```python
from build123d import *

# Parameters (mm, degrees)
SKETCH001_W        = 48
SKETCH001_H        = 51
SKETCH001_R        = 3.5
SKETCH001_R_2      = 2.25
PAD_DEPTH          = 3.41
SKETCH002_W        = 51
SKETCH002_H        = 45
PAD001_DEPTH       = 2.17
PAD002_DEPTH       = 25.56
POLARPATTERN_COUNT = 4
PAD003_DEPTH       = 3
CHAMFER_SIZE       = 2.8
FILLET_R           = 6
FILLET001_R        = 22


with BuildPart() as part:
    # Sketch001 → Pad (new body)
    with BuildSketch(Plane.XY):
        Rectangle(SKETCH001_W, SKETCH001_H)
        with Locations((-18.5, 17)):
            Circle(SKETCH001_R, mode=Mode.SUBTRACT)
        with Locations((15, 17)):
            Circle(SKETCH001_R_2, mode=Mode.SUBTRACT)
        with Locations((-18.5, -17)):
            Circle(SKETCH001_R, mode=Mode.SUBTRACT)
        with Locations((15, -17)):
            Circle(SKETCH001_R_2, mode=Mode.SUBTRACT)
    extrude(amount=PAD_DEPTH)

    # Sketch002 → Pad001 (join)
    with BuildSketch(Plane(origin=(-24, 0, 0), x_dir=(0, -1, 0), z_dir=(-1, 0, 0))):
        with Locations((0, 22.5)):
            Rectangle(SKETCH002_W, SKETCH002_H)
    extrude(amount=PAD001_DEPTH)

    # Sketch → Pad002 (join)
    with BuildSketch(Plane(origin=(-26.17, 0, 26), x_dir=(0, -1, 0), z_dir=(-1, 0, 0))):
        with BuildLine():
            ThreePointArc((16.420739, 4.399924), (12.028925, 12.0127), (4.422085, 16.414785))
            ThreePointArc((3.11174, 17.647793), (3.652144, 16.909322), (4.422085, 16.414785))
            ThreePointArc((3.11174, 17.647793), (2.656255, 18.151957), (2, 18.327959))
            ThreePointArc((2, 18.327959), (0, 18.53), (-2, 18.327959))
            ThreePointArc((-2, 18.327959), (-2.656255, 18.151957), (-3.11174, 17.647793))
            ThreePointArc((-4.400695, 16.423616), (-3.643735, 16.917271), (-3.11174, 17.647793))
            Line((-4.400695, 16.423616), (-3.882286, 14.488887))
            ThreePointArc((-2.03, 14.862002), (-2.962024, 14.704639), (-3.882286, 14.488887))
            Line((-2.03, 16.878362), (-2.03, 14.862002))
            ThreePointArc((2.03, 16.878362), (0, 17), (-2.03, 16.878362))
            Line((2.03, 16.878362), (2.03, 14.862002))
            ThreePointArc((14.488887, 3.882286), (9.917507, 11.253579), (2.03, 14.862002))
            Line((14.488887, 3.882286), (16.420739, 4.399924))
        make_face()
    pad002 = extrude(amount=PAD002_DEPTH)

    # PolarPattern: Pad002 ×4 about axis
    polarpattern_axis = Axis((-26.17, 0, 26), (-1, 0, 0))
    for i in range(1, POLARPATTERN_COUNT):
        add(pad002.rotate(polarpattern_axis, i * 360 / POLARPATTERN_COUNT))

    # Sketch003 → Pad003 (join)
    with BuildSketch(Plane.XZ.offset(-10)):
        with BuildLine():
            ThreePointArc((-24, 37.77), (-5.775752, 15.754927), (20, 3.41))
            Line((20, 3.41), (-24, 3.41))
            Line((-24, 3.41), (-24, 37.77))
        make_face()
    pad003 = extrude(amount=PAD003_DEPTH)

    # Mirrored: Pad003 across XZ
    add(pad003.mirror(Plane.XZ))

    # Chamfer
    chamfer_edges = [part.edges().sort_by_distance(p)[0] for p in [
        (12.75, 17, 3.41),
        (12.75, -17, 3.41),
    ]]
    chamfer(chamfer_edges, length=CHAMFER_SIZE)

    # Fillet
    fillet_edges = [part.edges().sort_by_distance(p)[0] for p in [
        (24, 25.5, 1.705),
        (24, -25.5, 1.705),
    ]]
    fillet(fillet_edges, radius=FILLET_R)

    # Fillet001
    fillet001_edges = [part.edges().sort_by_distance(p)[0] for p in [
        (-25.085, 25.5, 45),
        (-25.085, -25.5, 45),
    ]]
    fillet(fillet001_edges, radius=FILLET001_R)


solid = part.part
```
The model under review builds one solid part; all positions refer to its coordinate system, in mm. A direction names the side the tool comes from. Round coordinates to 2 decimals unless told otherwise and drop trailing zeros. Loops run counter-clockwise (first coordinate to the right, second up) from the corner with the lowest first, then second, coordinate; pieces in that order, holes last.
Item 1: Take a section at D-D (y = 0.5). Write out the cut boundary in (x, z).
Determined:
outline: (-51.73, 7.48) - (-26.17, 7.48) - (-26.17, 0) - (24, 0) - (24, 3.41) - (-24, 3.41) - (-24, 45) - (-26.17, 45) - (-26.17, 44.52) - (-51.73, 44.52) - (-51.73, 42.99) - (-26.17, 42.99) - (-26.17, 9.01) - (-51.73, 9.01) - close
Item 2: Take a section at B-B (z = 39). Write out the cut boundary in (x, y).
Determined:
outline: (-51.73, -10.95) - (-26.17, -10.95) - (-26.17, -18.6) - (-24, -18.6) - (-24, 18.6) - (-26.17, 18.6) - (-26.17, 10.95) - (-51.73, 10.95) - (-51.73, 7.48) - (-26.17, 7.48) - (-26.17, -7.48) - (-51.73, -7.48) - close
Item 3: For faces 1 (the face through (-39, 0, 43)), 2 (the face through (-38.77, -18.53, 25.97)), 3 (the face through (-12, 7, 13)), list the 3-axis set-ups (+Z, -Z, +X, -X, +Y, -Y) from which the entire face can be reached by the end or side of a thin tool; tool diameter is ignored.
Determined:
face 1: -X
face 2: -X, -Y
face 3: +Z, +X
Item 4: Clearance check with flat-ended pins moving along their axes: pin 1 Ø0.6 at (x, y) = (-38.5, -15.5) entering from -Z; pin 2 Ø4 at (x, z) = (-40, 21) entering from +Y; pin 3 Ø17 at (y, z) = (-1.5, 23) entering from -X. State where each tip first meets the part, or that it passes through.
Determined:
pin 1: stops at z = 18.39
pin 2: stops at y = 17.83
pin 3: stops at x = -26.17
Item 5: Take a section at C-C (x = 4). Write out the cut boundary in (y, z), then the cut area to 3 significant figures.
Determined:
outline: (-25.5, 0) - (25.5, 0) - (25.5, 3.41) - (10, 3.41) - (10, 9.41) - (7, 9.41) - (7, 3.41) - (-7, 3.41) - (-7, 9.41) - (-10, 9.41) - (-10, 3.41) - (-25.5, 3.41) - close
area: 210 mm2
Item 6: Mouldability with a two-part tool opening along X and no side actions: class faces 4 (the face through (13.107, 15.548, 0.746)), 5 (the face through (-16.62, 19.95, 1.68)), 6 (the face through (-6.09, 8.52, 16)), 7 (the face through (-12, -10, 13)) as released by +X, released by -X, zero draft, split by the parting line, or undercut.
Determined:
face 4: undercut
face 5: undercut
face 6: released by +X
face 7: zero draft
Item 7: Take a section at A-A (x = -16.5). Write out the cut boundary in (y, z).
Determined:
outline: (-25.5, 0) - (-19.87, 0) - (-19.87, 3.41) - (-25.5, 3.41) - close; (-14.13, 0) - (14.13, 0) - (14.13, 3.41) - (10, 3.41) - (10, 26.28) - (7, 26.28) - (7, 3.41) - (-7, 3.41) - (-7, 26.28) - (-10, 26.28) - (-10, 3.41) - (-14.13, 3.41) - close; (19.87, 0) - (25.5, 0) - (25.5, 3.41) - (19.87, 3.41) - close
Item 8: For line 1 (Y direction, x = 15, z = 0.2); line 2 (Y direction, x = -20.5, z = 11.5); line 3 (Z direction, x = -32, y = 10.5), list the stretches that pass through material, from the lowest coordinate up.
Determined:
line 1: y = -25.5 to -19.25, -14.75 to 14.75, 19.25 to 25.5
line 2: y = -10 to -7, 7 to 10
line 3: z = 12.63 to 15.29, 36.71 to 39.37
